The model under review builds one solid part; all positions refer to its coordinate system, in mm. Coordinates: 2 decimals unless noted, no trailing zeros. Write each loop counter-clockwise with the first axis right and the second up, starting at its lowest first coordinate (ties: lowest second). Pieces come first, ordered by that corner, then holes.
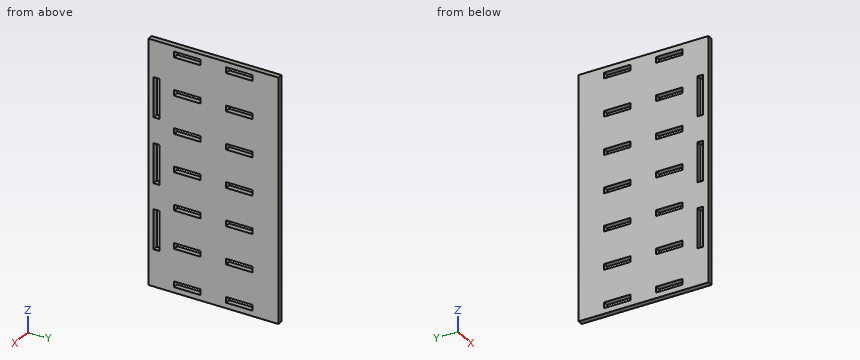
```python
from build123d import *

# Parameters (mm, degrees)
SKETCH_1_W      = 186.6
SKETCH_1_H      = 100
SKETCH_1_W_2    = 4.4
SKETCH_1_H_2    = 20.4
SKETCH_1_W_3    = 30.4
SKETCH_1_H_3    = 4.4
EXTRUDE_1_DEPTH = 4


with BuildPart() as part:
    # Эскиз1 → Бобышка-Вытянуть1 (new body)
    with BuildSketch(Plane(origin=(0, 0, 0), x_dir=(0, 0, -1), z_dir=(1, 0, 0))):
        with Locations((93.3, 50)):
            Rectangle(SKETCH_1_W, SKETCH_1_H)
        with Locations((6.2, 30)):
            Rectangle(SKETCH_1_W_2, SKETCH_1_H_2, mode=Mode.SUBTRACT)
        with Locations((6.2, 70)):
            Rectangle(SKETCH_1_W_2, SKETCH_1_H_2, mode=Mode.SUBTRACT)
        with Locations((35.2, 70)):
            Rectangle(SKETCH_1_W_2, SKETCH_1_H_2, mode=Mode.SUBTRACT)
        with Locations((35.2, 30)):
            Rectangle(SKETCH_1_W_2, SKETCH_1_H_2, mode=Mode.SUBTRACT)
        with Locations((64.2, 70)):
            Rectangle(SKETCH_1_W_2, SKETCH_1_H_2, mode=Mode.SUBTRACT)
        with Locations((64.2, 30)):
            Rectangle(SKETCH_1_W_2, SKETCH_1_H_2, mode=Mode.SUBTRACT)
        with Locations((93.2, 70)):
            Rectangle(SKETCH_1_W_2, SKETCH_1_H_2, mode=Mode.SUBTRACT)
        with Locations((93.2, 30)):
            Rectangle(SKETCH_1_W_2, SKETCH_1_H_2, mode=Mode.SUBTRACT)
        with Locations((122.2, 70)):
            Rectangle(SKETCH_1_W_2, SKETCH_1_H_2, mode=Mode.SUBTRACT)
        with Locations((122.2, 30)):
            Rectangle(SKETCH_1_W_2, SKETCH_1_H_2, mode=Mode.SUBTRACT)
        with Locations((151.2, 70)):
            Rectangle(SKETCH_1_W_2, SKETCH_1_H_2, mode=Mode.SUBTRACT)
        with Locations((151.2, 30)):
            Rectangle(SKETCH_1_W_2, SKETCH_1_H_2, mode=Mode.SUBTRACT)
        with Locations((180.2, 70)):
            Rectangle(SKETCH_1_W_2, SKETCH_1_H_2, mode=Mode.SUBTRACT)
        with Locations((180.2, 30)):
            Rectangle(SKETCH_1_W_2, SKETCH_1_H_2, mode=Mode.SUBTRACT)
        with Locations((43.2, 6.2)):
            Rectangle(SKETCH_1_W_3, SKETCH_1_H_3, mode=Mode.SUBTRACT)
        with Locations((93.2, 6.2)):
            Rectangle(SKETCH_1_W_3, SKETCH_1_H_3, mode=Mode.SUBTRACT)
        with Locations((143.2, 6.2)):
            Rectangle(SKETCH_1_W_3, SKETCH_1_H_3, mode=Mode.SUBTRACT)
    extrude(amount=EXTRUDE_1_DEPTH)


solid = part.part
```
Item 1: Take a section at B-B, the plane y = 38. Count the separate pieces of the cut face and the enclosed holes in it, plus the area to 3 significant figures.
Solved:
separate pieces: 8
enclosed holes: 0
area: 623 mm2
Item 2: To check wall thickness, follow line 1 along Y through (x, z) = (1.15, -121.5); line 2 along Y through (x, z) = (3.2, -92); line 3 along Y through (x, z) = (2.4, -158). State the ranges of each line that lie inside material, in increasing order.
Solved:
line 1: y = 0 to 19.8, 40.2 to 59.8, 80.2 to 100
line 2: y = 0 to 4, 8.4 to 19.8, 40.2 to 59.8, 80.2 to 100
line 3: y = 0 to 4, 8.4 to 100
Item 3: Take a section at A-A, the plane z = -87.5. Write out the cut boundary in (x, y), plus the area to 3 significant figures.
Solved:
outline: (0, 0) - (4, 0) - (4, 4) - (0, 4) - close; (0, 8.4) - (4, 8.4) - (4, 100) - (0, 100) - close
area: 382 mm2
